from build123d import *

# Parameters (mm, degrees)
BODYSKE_R  = 1.7272
BODY_DEPTH = 9.4234


with BuildPart() as part:
    # BodySke → Body (new body)
    with BuildSketch(Plane(origin=(0, 0, 0), x_dir=(0, 0, -1), z_dir=(1, 0, 0))):
        with BuildLine():
            Line((-5.8928, -9.525), (5.8928, -9.525))
            Line((5.8928, -9.525), (5.8928, -8.9154))
            Line((5.8928, -8.9154), (4.842933333, -8.9154))
            Line((4.842933333, -8.9154), (4.842933333, -8.6106))
            Line((4.842933333, -8.6106), (5.1054, -8.6106))
            Line((5.1054, -8.6106), (5.1054, -8.001))
            Line((5.1054, -8.001), (4.504485143, -6.35))
            Line((4.504485143, -6.35), (3.520438226, -6.35))
            ThreePointArc((3.520438226, -6.35), (2.069125842, -5.296760115), (2.620488612, -3.59041285))
            ThreePointArc((2.620488612, -3.59041285), (0, 4.445), (-2.620488612, -3.59041285))
            ThreePointArc((-2.620488612, -3.59041285), (-2.069125842, -5.296760115), (-3.520438226, -6.35))
            Line((-3.520438226, -6.35), (-4.504485143, -6.35))
            Line((-4.504485143, -6.35), (-5.1054, -8.001))
            Line((-5.1054, -8.001), (-5.1054, -8.6106))
            Line((-5.1054, -8.6106), (-4.842933333, -8.6106))
            Line((-4.842933333, -8.6106), (-4.842933333, -8.9154))
            Line((-4.842933333, -8.9154), (-5.8928, -8.9154))
            Line((-5.8928, -8.9154), (-5.8928, -9.525))
        make_face()
        Circle(BODYSKE_R, mode=Mode.SUBTRACT)
    extrude(amount=BODY_DEPTH)

    # EndChamferSke → EndChamfer (revolve, cut)
    with BuildSketch(Plane.XY, mode=Mode.PRIVATE) as endchamfer_sk:
        Polygon((-0.254, 2.0828), (0.00254, 2.0828), (0.251441319, 1.7272), (-0.254, 1.7272), align=None)
        Polygon((9.6774, 2.0828), (9.42086, 2.0828), (9.171958681, 1.7272), (9.6774, 1.7272), align=None)
    revolve(endchamfer_sk.sketch.rotate(Axis((-5.105879624, 0, 0), (1, 0, 0)), 90), axis=Axis((-5.105879624, 0, 0), (1, 0, 0)), mode=Mode.SUBTRACT)


solid = part.part
Input: part model. Units: mm. Frame: model coordinates. A direction names the side the tool comes from. Give positions to 0.01 mm unless a question says otherwise; leave off trailing zeros. Loops run counter-clockwise (first coordinate to the right, second up) from the corner with the lowest first, then second, coordinate; pieces in that order, holes last. Notation, with made-up numbers: M -18.5,-15 L 39.5,-15 A23 cw 39.5,1 Z; hole C -15,42 d3. An arc over 180 degrees is marked long. Use CSV: the item, a comma, the result in double quotes.
(1) Pin query (flat end, axial travel): P1, Ø0.5, axis at x = 6.5, y = -8.5, coming from the +Z side; P2, Ø4, axis at x = 3, y = 1, coming from the +Z side (3 decimals); P3, Ø0.8, axis at x = 6.5, z = 4, coming from the +Y side. Return the tip coordinate at first contact, or that it passes through.
Outcome:
P1,"stops at z = 5.11"
P2,"stops at z = 4.445"
P3,"stops at y = 2.61"
(2) Set-up query: faces 4 (the face through (5, -6.35, -4)), 5 (the face through (4.646, 4.442, -0.156)), 6 (the face through (5, -8.915, 5)). Return all of +Z, -Z, +X, -X, +Y, -Y with unobstructed straight access to the full face (end or side cutting, diameter ignored); none if empty.
Outcome:
face 4,"-Z, +X, -X"
face 5,"+X, -X"
face 6,"+Z, +X, -X"
(3) Section D-D, the plane z = 3.75. Return loops of the section in (x, y) (3 decimals).
Outcome:
outline,"M 0,-9.525 L 9.423,-9.525 L 9.423,-6.35 L 0,-6.35 Z; M 0,-2.387 L 9.423,-2.387 L 9.423,2.387 L 0,2.387 Z"
(4) Material intervals for L1, parallel to Y at x = 5.5, z = 3 (3 decimals); L2, parallel to Z at x = 3.5, y = -0.5; L3, parallel to Z at x = 1.25, y = -8.5, sorted ascending. Write a range as [from, to].
Outcome:
L1,"y = [-9.525, -6.259], [-3.28, 3.28]"
L2,"z = [-4.42, -1.65], [1.65, 4.42]"
L3,"z = [-5.11, 5.11]"
(5) Section C-C, the plane x = 0.5. Return loops of the section in (y, z) (3 decimals).
Outcome:
outline,"M -9.525,-5.893 L -8.915,-5.893 L -8.915,-4.843 L -8.611,-4.843 L -8.611,-5.105 L -8.001,-5.105 L -6.35,-4.504 L -6.35,-3.52 A1.527 cw -3.59,-2.62 A4.445 ccw long -3.59,2.62 A1.527 cw -6.35,3.52 L -6.35,4.504 L -8.001,5.105 L -8.611,5.105 L -8.611,4.843 L -8.915,4.843 L -8.915,5.893 L -9.525,5.893 Z; hole C 0,0 d3.454"
(6) Pull-direction query (Z, two-part tool) for faces 1 (the face through (4.649, 1.713, 0.225)), 2 (the face through (5, -6.35, 4)), 3 (the face through (4.65, -7.19, -4.81)); classes: pulls with the +Z half, pulls with the -Z half, needs draft (parallel to the pull), parting line crosses it, or undercut.
Outcome:
face 1,"undercut"
face 2,"needs draft"
face 3,"pulls with the -Z half"
